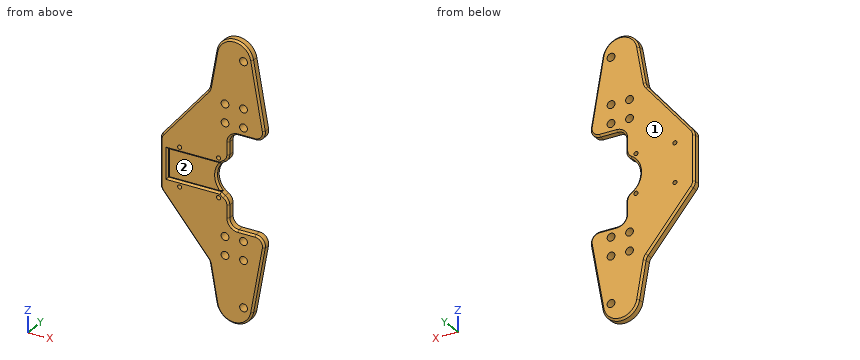
from build123d import *

# Parameters (mm, degrees)
EXTRUDE_1_DEPTH          = 2.5
SKETCH_2_R               = 2.1
CUT_EXTRUDE_1_DEPTH      = 86.14693183
SKETCH_3_R               = 1.1
CUT_EXTRUDE_2_DEPTH      = 86.14693183
SKETCH_6_W               = 36
SKETCH_6_H               = 15
CUT_EXTRUDE_3_DEPTH      = 1.5
CHAMFER_1_SIZE           = 1
CUT_EXTRUDE_4_DEPTH      = 86.14693183
CUT_EXTRUDE_4_DEPTH_BACK = 86.14693183
SKETCH_7_R               = 2.1


with BuildPart() as part:
    # 草图1 → 凸台-拉伸1 (new, symmetric)
    with BuildSketch(Plane(origin=(0, 0, 0), x_dir=(1, 0, 0), z_dir=(0, 1, 0))):
        with BuildLine():
            Line((16.172616149, -30.868240888), (9.84807753, -66.736481777))
            ThreePointArc((9.84807753, -66.736481777), (0, -75), (-9.84807753, -66.736481777))
            Line((-9.84807753, -66.736481777), (-13.366457523, -46.782757288))
            ThreePointArc((-13.366457523, -46.782757288), (-13.758957353, -45.537906868), (-14.460274073, -44.437060128))
            Line((-14.460274073, -44.437060128), (-38.830222216, -15.394086877))
            ThreePointArc((-38.830222216, -15.394086877), (-39.698463104, -13.890249545), (-40, -12.180148829))
            Line((-40, -12.180148829), (-40, 12.180148829))
            ThreePointArc((-40, 12.180148829), (-39.698463104, 13.890249545), (-38.830222216, 15.394086877))
            Line((-38.830222216, 15.394086877), (-14.460274073, 44.437060128))
            ThreePointArc((-14.460274073, 44.437060128), (-13.758957353, 45.537906868), (-13.366457523, 46.782757288))
            Line((-13.366457523, 46.782757288), (-9.84807753, 66.736481777))
            ThreePointArc((-9.84807753, 66.736481777), (0, 75), (9.84807753, 66.736481777))
            Line((9.84807753, 66.736481777), (16.172616149, 30.868240888))
            ThreePointArc((16.172616149, 30.868240888), (15.0787996, 26.786061952), (11.248577384, 25))
            Line((11.248577384, 25), (2, 25))
            ThreePointArc((2, 25), (-1.535533906, 23.535533906), (-3, 20))
            Line((-3, 20), (-3, 13.275918047))
            ThreePointArc((-3, 13.275918047), (-3.646654975, 10.816571163), (-5.419354839, 8.993363839))
            ThreePointArc((-5.419354839, 8.993363839), (-10.5, 0), (-5.419354839, -8.993363839))
            ThreePointArc((-5.419354839, -8.993363839), (-3.646654975, -10.816571163), (-3, -13.275918047))
            Line((-3, -13.275918047), (-3, -20))
            ThreePointArc((-3, -20), (-1.535533906, -23.535533906), (2, -25))
            Line((2, -25), (11.248577384, -25))
            ThreePointArc((11.248577384, -25), (15.0787996, -26.786061952), (16.172616149, -30.868240888))
        make_face()
    extrude(amount=EXTRUDE_1_DEPTH, both=True)

    # 草图2 → 切除-拉伸1 (cut, through all)
    with BuildSketch(Plane(origin=(0, 2.5, 0), x_dir=(1, 0, 0), z_dir=(0, 1, 0))):
        with Locations(Location((5, -65, 0), (0, 0, 270))):
            Circle(SKETCH_2_R)
        with Locations(Location((5, 65, 0), (0, 0, 90))):
            Circle(SKETCH_2_R)
    extrude(amount=-CUT_EXTRUDE_1_DEPTH, mode=Mode.SUBTRACT)

    # 草图3 → 切除-拉伸2 (cut, through all)
    with BuildSketch(Plane.XZ.offset(2.5)):
        with Locations(Location((-8.5, 10.5, 0), (0, 0, 270))):
            Circle(SKETCH_3_R)
        with Locations(Location((-29.5, 10.5, 0), (0, 0, 270))):
            Circle(SKETCH_3_R)
        with Locations(Location((-29.5, -10.5, 0), (0, 0, 90))):
            Circle(SKETCH_3_R)
        with Locations(Location((-8.5, -10.5, 0), (0, 0, 90))):
            Circle(SKETCH_3_R)
    extrude(amount=-CUT_EXTRUDE_2_DEPTH, mode=Mode.SUBTRACT)

    # 草图6 → 切除-拉伸3 (cut)
    with BuildSketch(Plane.XZ.offset(2.5)):
        with Locations((-18, 0)):
            Rectangle(SKETCH_6_W, SKETCH_6_H)
    extrude(amount=-CUT_EXTRUDE_3_DEPTH, mode=Mode.SUBTRACT)

    # 倒角1
    chamfer_1_edges = [part.edges().sort_by_distance(p)[0] for p in [
        (-6.427430804, -2.5, -8.302899088),
        (-21.674234614, -2.5, 7.5),
        (-10.5, -1, 0),
        (-36, -2.5, 0),
        (-21.674234614, -2.5, -7.5),
        (-1.535533906, 2.5, 23.535533906),
        (-3, 2.5, 16.637959024),
        (-3.646654975, 2.5, 10.816571163),
        (13.01034684, -2.5, 48.802361333),
        (0, -2.5, 75),
        (-11.607267527, -2.5, 56.759619532),
        (-13.758957353, -2.5, 45.537906868),
        (-26.645248144, -2.5, 29.915573502),
        (-10.5, 2.5, 0),
        (-39.698463104, -2.5, 13.890249545),
        (-40, -2.5, 0),
        (-39.698463104, -2.5, -13.890249545),
        (-26.645248144, -2.5, -29.915573502),
        (-13.758957353, -2.5, -45.537906868),
        (-11.607267527, -2.5, -56.759619532),
        (0, -2.5, -75),
        (13.01034684, -2.5, -48.802361333),
        (15.0787996, -2.5, -26.786061952),
        (6.624288692, -2.5, -25),
        (-3.646654975, 2.5, -10.816571163),
        (-1.535533906, -2.5, -23.535533906),
        (-3, -2.5, -16.637959024),
        (-3.646654975, -2.5, -10.816571163),
        (-6.427430804, -2.5, 8.302899088),
        (-3.646654975, -2.5, 10.816571163),
        (-3, -2.5, 16.637959024),
        (-1.535533906, -2.5, 23.535533906),
        (6.624288692, -2.5, 25),
        (15.0787996, -2.5, 26.786061952),
        (-3, 2.5, -16.637959024),
        (-1.535533906, 2.5, -23.535533906),
        (6.624288692, 2.5, -25),
        (15.0787996, 2.5, -26.786061952),
        (13.01034684, 2.5, -48.802361333),
        (15.0787996, 2.5, 26.786061952),
        (0, 2.5, -75),
        (-11.607267527, 2.5, -56.759619532),
        (-13.758957353, 2.5, -45.537906868),
        (-26.645248144, 2.5, -29.915573502),
        (-39.698463104, 2.5, -13.890249545),
        (-40, 2.5, 0),
        (-39.698463104, 2.5, 13.890249545),
        (-26.645248144, 2.5, 29.915573502),
        (-13.758957353, 2.5, 45.537906868),
        (-11.607267527, 2.5, 56.759619532),
        (6.624288692, 2.5, 25),
        (0, 2.5, 75),
        (13.01034684, 2.5, 48.802361333),
    ]]
    chamfer(chamfer_1_edges, length=CHAMFER_1_SIZE)

    # 草图7 → 切除-拉伸4 (cut, two sides: drawn at the far end of the back side and taken through both)
    with BuildSketch(Plane(origin=(0, 2.5, 0), x_dir=(1, 0, 0), z_dir=(0, 1, 0)).offset(-CUT_EXTRUDE_4_DEPTH_BACK)):
        with Locations(Location((-5, 40, 0), (0, 0, 270))):
            Circle(SKETCH_7_R)
        with Locations(Location((5, 40, 0), (0, 0, 270))):
            Circle(SKETCH_7_R)
        with Locations(Location((5, -40, 0), (0, 0, 90))):
            Circle(SKETCH_7_R)
        with Locations(Location((-5, -40, 0), (0, 0, 90))):
            Circle(SKETCH_7_R)
        with Locations(Location((-5, 30, 0), (0, 0, 270))):
            Circle(SKETCH_7_R)
        with Locations(Location((5, 30, 0), (0, 0, 270))):
            Circle(SKETCH_7_R)
        with Locations(Location((5, -30, 0), (0, 0, 90))):
            Circle(SKETCH_7_R)
        with Locations(Location((-5, -30, 0), (0, 0, 90))):
            Circle(SKETCH_7_R)
    extrude(amount=CUT_EXTRUDE_4_DEPTH + CUT_EXTRUDE_4_DEPTH_BACK, mode=Mode.SUBTRACT)


solid = part.part
Could you check a few things on this model? Use its own coordinates, in mm. Face numbers are marked on the shaded views. Coordinates: 2 decimals unless noted, no trailing zeros. Loops run counter-clockwise (first coordinate to the right, second up) from the corner with the lowest first, then second, coordinate; pieces in that order, holes last.
1. Imagine slicing it at B-B (x = -24). Please give me the cut outline in (y, z).
2. Imagine slicing it at D-D (x = 5). Give the number of separate pieces and of enclosed holes in the cut face, and give its area (3 significant figures).
3. For P1, Ø7.5, axis at x = -18.5, z = 1.5, coming from the -Y side; P2, Ø2, axis at y = -0.5, z = 32.5, coming from the +X side; P3, Ø2, axis at x = -8.5, z = -10.5, coming from the -Y side; P4, Ø1.7, axis at x = -17.5, y = -0.5, coming from the +Z side, each with a flat end and sliding along its axis, tell me the tip position at first contact or that it passes through.
4. We'd pull the mould along Z, two halves only. Please class the marked faces 1 and 2: released by +Z, released by -Z, zero draft, split by the parting line, or undercut.
5. Imagine slicing it at C-C (z = 17). Please give me the cut outline in (x, y).
6. I need wall thicknesses on L1, parallel to Z at x = -3.5, y = 0.3; L2, parallel to X at y = -0.1, z = -30; L3, parallel to X at y = -1.05, z = 41. Which ranges of each line are inside material? Lowest first, please.
7. Imagine slicing it at A-A (z = -65). Please give me the cut outline in (x, y).
Computed values:
1. outline: (-2.5, -31.51) - (-1.5, -33.07) - (1.5, -33.07) - (2.5, -31.51) - (2.5, 31.51) - (1.5, 33.07) - (-1.5, 33.07) - (-2.5, 31.51) - (-2.5, 8.5) - (-1.5, 7.5) - (-1, 7.5) - (-1, -7.5) - (-1.5, -7.5) - (-2.5, -8.5) - close
2. separate pieces: 8
2. enclosed holes: 0
2. area: 356 mm2
3. P1: stops at y = -1
3. P2: stops at x = 16.06
3. P3: passes through
3. P4: stops at z = 41.83
4. face 1: zero draft
4. face 2: undercut
5. outline: (-37.48, -1.5) - (-36.18, -2.5) - (-4, -2.5) - (-3, -1.5) - (-3, 1.5) - (-4, 2.5) - (-36.18, 2.5) - (-37.48, 1.5) - close
6. L1: z = -74.37 to -41.47, -38.53 to -31.47, -28.53 to -11.1, 11.1 to 28.53, 31.47 to 38.53, 41.47 to 74.37
6. L2: x = -26.57 to -7.1, -2.9 to 2.9, 7.1 to 16.25
6. L3: x = -17.34 to -6.85, -3.15 to 3.15, 6.85 to 14.39
7. outline: (-10.15, -1.5) - (-9.14, -2.5) - (2.9, -2.5) - (2.9, 2.5) - (-9.14, 2.5) - (-10.15, 1.5) - close; (7.1, -2.5) - (9.14, -2.5) - (10.15, -1.5) - (10.15, 1.5) - (9.14, 2.5) - (7.1, 2.5) - close
